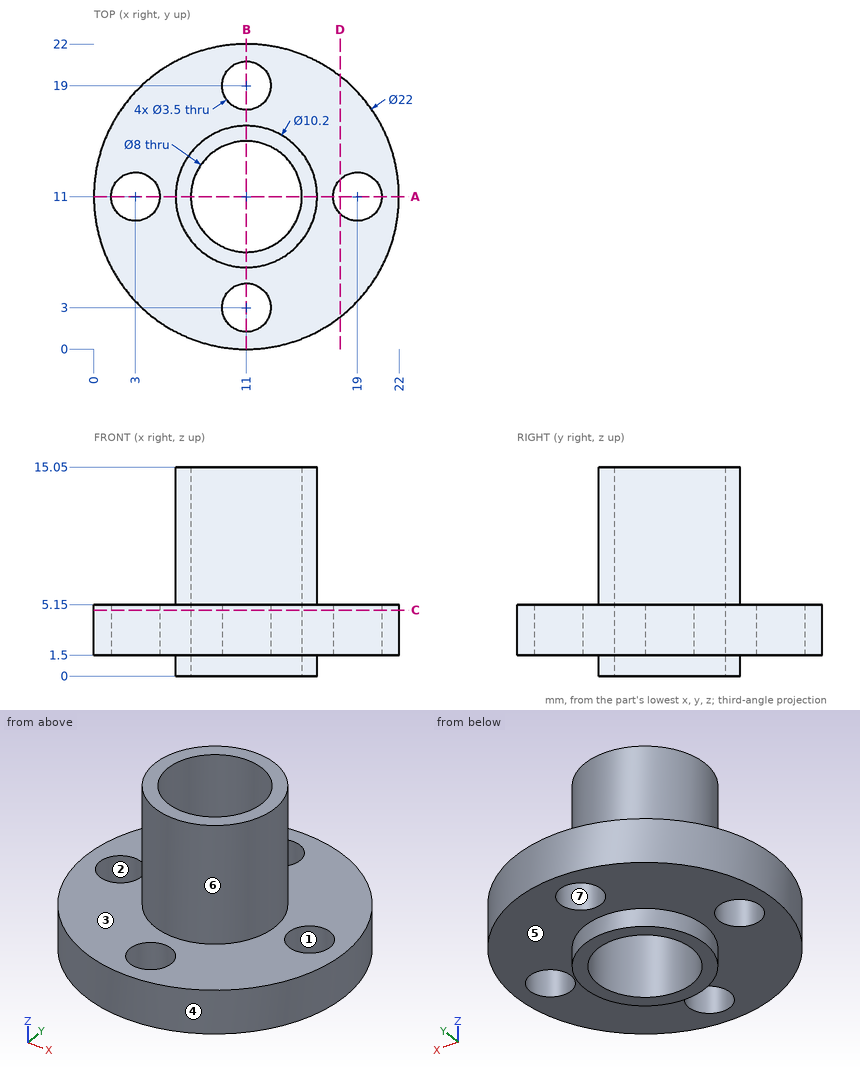
Job drawing, mm, ordinate dimensions from the low corner. One solid piece. A direction names the side the tool comes from. Round coordinates to 2 decimals unless told otherwise and drop trailing zeros. Loops run counter-clockwise (first coordinate to the right, second up) from the corner with the lowest first, then second, coordinate; pieces in that order, holes last. Notation, with made-up numbers: (72, 22) -> (81, 22) arc R17 ccw to (81, 44) -> close; hole circle Ø9 at (-26.75, 83). An arc over 180 degrees is marked (long way). Use CSV: the item, a comma, the result in double quotes. Start each with the question number.
Q1. Drill centre lines: L1, parallel to Y at x = 11, z = 3.6; L2, parallel to X at y = 11, z = 8.5. Where is each one in solid material? Low to high.
Q2. Flat gauge pins, fed straight in: pin 1 Ø1 at (x, z) = (17, 3) entering from +Y; pin 2 Ø8 at (x, z) = (15.5, 3) entering from +Y; pin 3 Ø5.5 at (x, y) = (11, 19) entering from -Z; pin 4 Ø3 at (x, y) = (3, 11) entering from +Z. Where does each tip first touch, or does it go through?
Q3. Saw through at D-D on x = 17.75. Give the cut face in (y, z).
Q4. Saw through at C-C on z = 4.75. Give the cut face in (x, y).
Q5. Mould opens along X. For the marked faces 1, 2, 3 and 4 say: +X half, -X half, draft (parallel to the pull), parting line (faces both ways), or undercut.
Q6. Saw through at A-A on y = 11. Give the cut face in (x, z).
Q7. Which spindle directions (+Z, -Z, +X, -X, +Y, -Y) get a long thin tool onto all of the face, cutting with end or side? Do the marked faces 5, 6 and 7. Say none if no direction does.
Solutions:
1,L1,"y = 0 to 1.25, 4.75 to 7, 15 to 17.25, 20.75 to 22"
1,L2,"x = 5.9 to 7, 15 to 16.1"
2,pin 1,"stops at y = 20.53"
2,pin 2,"stops at y = 21.99"
2,pin 3,"stops at z = 1.5"
2,pin 4,"passes through"
3,outline,"(2.31, 1.5) -> (9.78, 1.5) -> (9.78, 5.15) -> (2.31, 5.15) -> close; (12.22, 1.5) -> (19.69, 1.5) -> (19.69, 5.15) -> (12.22, 5.15) -> close"
4,outline,"circle Ø22 at (11, 11); hole circle Ø3.5 at (3, 11); hole circle Ø8 at (11, 11); hole circle Ø3.5 at (11, 3); hole circle Ø3.5 at (11, 19); hole circle Ø3.5 at (19, 11)"
5,face 1,"undercut"
5,face 2,"undercut"
5,face 3,"draft"
5,face 4,"parting line"
6,outline,"(0, 1.5) -> (1.25, 1.5) -> (1.25, 5.15) -> (0, 5.15) -> close; (4.75, 1.5) -> (5.9, 1.5) -> (5.9, 0) -> (7, 0) -> (7, 15.05) -> (5.9, 15.05) -> (5.9, 5.15) -> (4.75, 5.15) -> close; (15, 0) -> (16.1, 0) -> (16.1, 1.5) -> (17.25, 1.5) -> (17.25, 5.15) -> (16.1, 5.15) -> (16.1, 15.05) -> (15, 15.05) -> close; (20.75, 1.5) -> (22, 1.5) -> (22, 5.15) -> (20.75, 5.15) -> close"
7,face 5,"-Z"
7,face 6,"+Z"
7,face 7,"+Z, -Z"
